Can you work these out from the model? Positions are in its coordinate system, mm. Give positions to 0.01 mm unless a question says otherwise; leave off trailing zeros. Loops run counter-clockwise (first coordinate to the right, second up) from the corner with the lowest first, then second, coordinate; pieces in that order, holes last. Notation, with made-up numbers: (44, 64) - (75, 64) arc R24 ccw to (75, 83) - close; hole circle Ø5 at (0.5, -17). An arc over 180 degrees is marked (long way). Use a Markdown table: item, result. Add a question column.
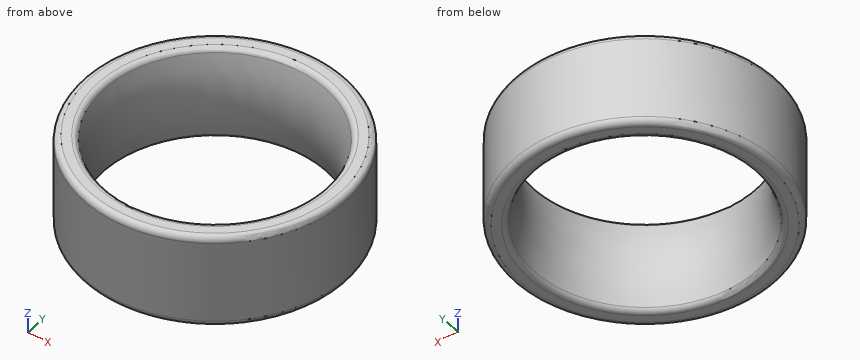
```python
from build123d import *


with BuildPart() as f1:
    # F0 (on Front) → F1 (revolve)
    with BuildSketch(Plane.XZ):
        with BuildLine():
            ThreePointArc((-9.3945671041, 7.608697411), (-9.5809203898, 7.8472895911), (-9.8699114928, 7.9375))
            Line((-9.8699114928, 7.9375), (-10.6045, 7.9375))
            ThreePointArc((-10.6045, 7.9375), (-10.9637102448, 7.7887102448), (-11.1125, 7.4295))
            Line((-11.1125, 7.4295), (-11.1125, 0.508))
            ThreePointArc((-11.1125, 0.508), (-10.9637102448, 0.1487897552), (-10.6045, 0))
            Line((-10.6045, 0), (-9.8699114928, 0))
            ThreePointArc((-9.8699114928, 0), (-9.5809203898, 0.0902104089), (-9.3945671041, 0.328802589))
            ThreePointArc((-9.3945671041, 0.328802589), (-8.73125, 3.96875), (-9.3945671041, 7.608697411))
        make_face()
    revolve(axis=Axis((0, 0, 3.96875), (0, 0, 1)))


solid = f1.part
```
1. Suppose I cut it at D-D (z = 1.75). List the corners of the cut face in (x, y) for me (1 decimal), and give its area (3 significant figures).
2. Suppose I cut it at C-C (z = 6.25). List the corners of the cut face in (x, y) for me (1 decimal).
3. Suppose I cut it at A-A (x = 0). List the corners of the cut face in (y, z) for me.
4. Please list where these lines run through material, in increasing order: line 1 along X through (y, z) = (-7, 6); line 2 along X through (y, z) = (4.25, 6.5); line 3 along Y through (x, z) = (5, 2). Write a range as [from, to].
5. Will these pins go through, and if not, where does the flat tip stop? P1, Ø4, axis at x = -7, y = -5, coming from the -Z side; P2, Ø1, axis at y = -6, z = 3.5, coming from the -X side; P3, Ø2, axis at x = 7, z = 2, coming from the -Y side; P4, Ø2, axis at y = 4, z = 6.5, coming from the -X side.
Results below:
| question | item | result |
|---|---|---|
| 1 | outline | circle Ø22.2 at (0, 0); hole circle Ø17.9 at (0, 0) |
| 1 | area | 135 mm² |
| 2 | outline | circle Ø22.2 at (0, 0); hole circle Ø18 at (0, 0) |
| 3 | outline | (-11.11, 0.51) arc R0.51 ccw to (-10.6, 0) - (-9.87, 0) arc R0.51 ccw to (-9.39, 0.33) arc R10.32 ccw to (-9.39, 7.61) arc R0.51 ccw to (-9.87, 7.94) - (-10.6, 7.94) arc R0.51 ccw to (-11.11, 7.43) - close; (9.39, 0.33) arc R0.51 ccw to (9.87, 0) - (10.6, 0) arc R0.51 ccw to (11.11, 0.51) - (11.11, 7.43) arc R0.51 ccw to (10.6, 7.94) - (9.87, 7.94) arc R0.51 ccw to (9.39, 7.61) arc R10.32 ccw to start |
| 4 | line 1 | [-8.63, -5.55], [5.55, 8.63] |
| 4 | line 2 | [-10.27, -7.99], [7.99, 10.27] |
| 4 | line 3 | [-9.92, -7.39], [7.39, 9.92] |
| 5 | P1 | z = 0 |
| 5 | P2 | x = -9.66 |
| 5 | P3 | y = -9.35 |
| 5 | P4 | x = -10.7 |
